```python
from build123d import *

# Parameters (mm, degrees)
PAD_DEPTH       = 76
POCKET_DEPTH    = 143.2
SKETCH002_W     = 40
SKETCH002_H     = 16
POCKET001_DEPTH = 44.801
POCKET002_DEPTH = 17.6
SKETCH004_R     = 10
POCKET003_DEPTH = 76.001


with BuildPart() as part:
    # Sketch → Pad (new body)
    with BuildSketch(Plane.XY):
        Polygon((-48, 44.8), (-48, 0), (-28, 0), (-28, 16), (28, 16), (28, 0), (48, 0), (48, 44.8), (28, 44.8), (28, 139.502577), (0, 188), (-28, 139.502577), (-28, 44.8), align=None)
    extrude(amount=PAD_DEPTH)

    # Sketch001 (on DatumPlane) → Pocket (cut)
    with BuildSketch(Plane.XZ.offset(-188)):
        Polygon((48, 76), (-48, 76), (-48, 0), (-28, 0), (-28, 44.8), (28, 44.8), (28, 0), (48, 0), align=None)
    extrude(amount=POCKET_DEPTH, mode=Mode.SUBTRACT)

    # Sketch002 (on Face7 of Pocket) → Pocket001 (cut, through all)
    with BuildSketch(Plane(origin=(0, 44.8, 0), x_dir=(-1, 0, 0), z_dir=(0, 1, 0))):
        with Locations((0, 68)):
            Rectangle(SKETCH002_W, SKETCH002_H)
    extrude(amount=-POCKET001_DEPTH, mode=Mode.SUBTRACT)

    # Sketch003 (on Face18 of Pocket001) → Pocket002 (cut)
    with BuildSketch(Plane.XY.offset(44.8)):
        Polygon((0, 188), (-17.551448, 157.6), (17.551448, 157.6), align=None)
    extrude(amount=-POCKET002_DEPTH, mode=Mode.SUBTRACT)

    # Sketch004 (on Face14 of Pocket002) → Pocket003 (cut, through all)
    with BuildSketch(Plane.YZ.offset(28)):
        with Locations((100, 22.4)):
            Circle(SKETCH004_R)
    extrude(amount=-POCKET003_DEPTH, mode=Mode.SUBTRACT)


solid = part.part
```
CAD build for the part. Positions are in the model's coordinates, mm. A direction names the side the tool comes from. Give positions to 0.01 mm unless a question says otherwise; leave off trailing zeros. Write each loop counter-clockwise with the first axis right and the second up, starting at its lowest first coordinate (ties: lowest second). Pieces come first, ordered by that corner, then holes. Notation, with made-up numbers: (-34.5, -39.75) -> (-25.5, -39.75) arc R18 cw to (-25.5, -15.75) -> close; hole circle Ø5 at (-32, -2.75). An arc over 180 degrees is marked (long way). Write each question's results on one line, items separated by ' | '.
1. Which spindle directions (+Z, -Z, +X, -X, +Y, -Y) get a long thin tool onto all of the face, cutting with end or side? Do faces 1 (the flat face through (-48, 23, 37)), 2 (the flat face through (-28, 8, 37)), 3 (the flat face through (0, 102, 44.8)), 4 (the flat face through (38, 0, 37)), 5 (the flat face through (-20, 31, 68)). Say none if no direction does.
Geometry check:
face 1: +Z, -Z, -X, +Y, -Y | face 2: +Z, -Z, -Y | face 3: +Z, +X, -X, +Y | face 4: +Z, -Z, +X, -X, -Y | face 5: +Z, +Y, -Y
2. Cut at D-D, the plane z = 66. Write the cut outline in (x, y).
Geometry check:
outline: (-48, 0) -> (-28, 0) -> (-28, 16) -> (-20, 16) -> (-20, 44.8) -> (-48, 44.8) -> close; (20, 16) -> (28, 16) -> (28, 0) -> (48, 0) -> (48, 44.8) -> (20, 44.8) -> close
3. Cut at A-A, the plane z = 22.4. Write the cut outline in (x, y).
Geometry check:
outline: (-48, 0) -> (-28, 0) -> (-28, 16) -> (28, 16) -> (28, 0) -> (48, 0) -> (48, 44.8) -> (28, 44.8) -> (28, 90) -> (-28, 90) -> (-28, 44.8) -> (-48, 44.8) -> close; (-28, 110) -> (28, 110) -> (28, 139.5) -> (0, 188) -> (-28, 139.5) -> close
4. Cut at B-B, the plane y = 100. Write the cut outline in (x, z), then the cut area to 3 significant figures.
Geometry check:
outline: (-28, 0) -> (28, 0) -> (28, 12.4) -> (-28, 12.4) -> close; (-28, 32.4) -> (28, 32.4) -> (28, 44.8) -> (-28, 44.8) -> close | area: 1,390 mm²
5. Two-plate mould, pull along X, no slides. Class faces 6 (the flat face through (0, 16, 29)), 7 (the flat face through (-28, 93, 32)), 8 (the flat face through (-1, 74, 0)), 9 (the flat face through (28, 8, 37)): pulls with the +X half, pulls with the -X half, needs draft (parallel to the pull), parting line crosses it, or undercut.
Geometry check:
face 6: undercut | face 7: pulls with the -X half | face 8: needs draft | face 9: undercut
6. Cut at C-C, the plane x = 22. Write the cut outline in (y, z).
Geometry check:
outline: (16, 0) -> (149.89, 0) -> (149.89, 44.8) -> (44.8, 44.8) -> (44.8, 76) -> (16, 76) -> close; hole circle Ø20 at (100, 22.4)
7. Drop flat-ended pins along their axis: P1, Ø2, axis at x = 16.5, z = 37.5, coming from the +Y side; P2, Ø4, axis at x = -32, z = 51, coming from the -Y side; P3, Ø4, axis at x = -3, z = 59, coming from the +Y side; P4, Ø15, axis at x = 7, y = 168.5, coming from the +Z side. Give the stop position or say it passes through.
Geometry check:
P1: y = 157.6 | P2: y = 0 | P3: y = 44.8 | P4: z = 27.2
8. Wall check: probe 1 along X at (y, z) = (9.5, 10); probe 2 along Z at (x, y) = (-3, 100); probe 3 along X at (y, z) = (38, 64). Give the ranges that are in metal, low to high. Write a range as [from, to].
Geometry check:
probe 1: [-48, -28], [28, 48] | probe 2: [0, 12.4], [32.4, 44.8] | probe 3: [-48, -20], [20, 48]
